from build123d import *

# Parameters (mm, degrees)
SKETCH3_R           = 48
BOSS_EXTRUDE2_DEPTH = 20
SKETCH4_W           = 25
SKETCH4_H           = 5
SKETCH4_H_2         = 10
BOSS_EXTRUDE4_DEPTH = 5
SKETCH5_W           = 20
SKETCH5_H           = 7
BOSS_EXTRUDE5_DEPTH = 6
SKETCH6_W           = 24
SKETCH6_H           = 19
BOSS_EXTRUDE6_DEPTH = 19
SKETCH7_R           = 7.15
CUT_EXTRUDE1_DEPTH  = 28
SKETCH8_W           = 3.5
SKETCH8_H           = 19
SKETCH8_W_2         = 7
CUT_EXTRUDE2_DEPTH  = 19


with BuildPart() as part:
    # Sketch3 → Boss-Extrude2 (new body)
    with BuildSketch(Plane(origin=(0, 0, 0), x_dir=(1, 0, 0), z_dir=(0, 1, 0))):
        with Locations(Location((0, 0, 0), (0, 0, 270))):
            Circle(SKETCH3_R)
    extrude(amount=BOSS_EXTRUDE2_DEPTH)

    # Sketch4 → Boss-Extrude4 (add)
    with BuildSketch(Plane(origin=(0, 20, 0), x_dir=(1, 0, 0), z_dir=(0, 1, 0))):
        with Locations((-19.905756196, -7.187203126)):
            Rectangle(SKETCH4_W, SKETCH4_H)
        with Locations((-19.905756196, -12.187203126)):
            Rectangle(SKETCH4_W, SKETCH4_H)
        with Locations((19.905756196, -9.687203126)):
            Rectangle(SKETCH4_W, SKETCH4_H_2)
    extrude(amount=BOSS_EXTRUDE4_DEPTH)

    # Sketch5 → Boss-Extrude5 (add)
    with BuildSketch(Plane(origin=(0, 25, 0), x_dir=(1, 0, 0), z_dir=(0, 1, 0))):
        with Locations((19.905756196, -9.687203126)):
            Rectangle(SKETCH5_W, SKETCH5_H)
        with Locations((-19.905756196, -9.687203126)):
            Rectangle(SKETCH5_W, SKETCH5_H)
    extrude(amount=BOSS_EXTRUDE5_DEPTH)

    # Sketch6 → Boss-Extrude6 (add)
    with BuildSketch(Plane(origin=(0, 20, 0), x_dir=(1, 0, 0), z_dir=(0, 1, 0))):
        with Locations((0, -36.5)):
            Rectangle(SKETCH6_W, SKETCH6_H)
        with Locations((0, 36.5)):
            Rectangle(SKETCH6_W, SKETCH6_H)
    extrude(amount=BOSS_EXTRUDE6_DEPTH)

    # Sketch7 → Cut-Extrude1 (cut)
    with BuildSketch(Plane(origin=(12, 0, 0), x_dir=(0, 0, -1), z_dir=(1, 0, 0))):
        with Locations((-36.5, 27.5)):
            Circle(SKETCH7_R)
        with Locations(Location((36.5, 27.5, 0), (0, 0, 180))):
            Circle(SKETCH7_R)
    extrude(amount=-CUT_EXTRUDE1_DEPTH, mode=Mode.SUBTRACT)

    # Sketch8 → Cut-Extrude2 (cut)
    with BuildSketch(Plane(origin=(0, 39, 0), x_dir=(1, 0, 0), z_dir=(0, 1, 0))):
        with Locations((-1.75, -36.5)):
            Rectangle(SKETCH8_W, SKETCH8_H)
        with Locations((1.75, -36.5)):
            Rectangle(SKETCH8_W, SKETCH8_H)
        with Locations((0, 36.5)):
            Rectangle(SKETCH8_W_2, SKETCH8_H)
    extrude(amount=-CUT_EXTRUDE2_DEPTH, mode=Mode.SUBTRACT)


solid = part.part
Can you work these out from the model? Positions are in its coordinate system, mm. A direction names the side the tool comes from. Coordinates: 2 decimals unless noted, no trailing zeros. Order: outer loops, then holes, each group sorted by start corner. A loop starts at its lowest first (then second) coordinate and runs counter-clockwise, first axis right, second up. Notation, with made-up numbers: M 14,-0.5 L 49,-0.5 A15 cw 49,19.5 Z; hole C 41.5,-3.75 d4. An arc over 180 degrees is marked long. Answer as CSV lines item,"result".
(1) Suppose I cut it at C-C on y = 27.5. Count the separate pieces of the cut face and the enclosed holes in it, plus the area to 3 significant figures.
Geometry check:
separate pieces,"10"
enclosed holes,"0"
area,"440 mm^2"
(2) Suppose I cut it at A-A on z = 34. Please give me the cut outline in (x, y), plus the area to 3 significant figures.
Geometry check:
outline,"M -33.88,0 L 33.88,0 L 33.88,20 L 12,20 L 12,20.8 L 3.5,20.8 L 3.5,20 L -3.5,20 L -3.5,20.8 L -12,20.8 L -12,20 L -33.88,20 Z; M -12,34.2 L -3.5,34.2 L -3.5,39 L -12,39 Z; M 3.5,34.2 L 12,34.2 L 12,39 L 3.5,39 Z"
area,"1,450 mm^2"
(3) I'm going to push flat-ended pins straight in: pin 1 (2 mm diameter, centred on x = -19, z = 8.5, fed in from +Y); pin 2 (1.5 mm diameter, centred on x = 1.5, y = 25.5, fed in from +Z); pin 3 (4 mm diameter, centred on x = 24, y = 23.5, fed in from -Z); pin 4 (2.5 mm diameter, centred on y = 22, z = 12, fed in from -X). Where does each tip first touch, or does it pass through?
Geometry check:
pin 1,"y = 31"
pin 2,"through"
pin 3,"z = 4.69"
pin 4,"x = -32.41"
(4) Suppose I cut it at B-B on x = 5.5. Please give me the cut outline in (y, z), plus the area to 3 significant figures.
Geometry check:
outline,"M 0,-47.68 L 20,-47.68 L 20,-46 L 39,-46 L 39,-27 L 20,-27 L 20,27 L 39,27 L 39,46 L 20,46 L 20,47.68 L 0,47.68 Z; hole C 27.5,-36.5 d14.3; hole C 27.5,36.5 d14.3"
area,"2,310 mm^2"
(5) On a 3-axis mill with a long thin cutter (end or side, diameter ignored), from which of +Z, -Z, +X, -X, +Y, -Y can I reach the whole of each face in a straight line? I mean faces 1 (the flat face through (-20, 22, 4.687)), 2 (the flat face through (8, 29, -46)), 3 (the flat face through (-29.906, 28, 10)). Say none if no direction works.
Geometry check:
face 1,"+X, -X, +Y"
face 2,"-Z, +X, -X, +Y"
face 3,"+Z, -Z, -X, +Y"
(6) Please list where these lines run through material, in increasing order: L1, parallel to Z at x = -9, y = 27; L2, parallel to Y at x = 6, z = -36.5; L3, parallel to X at y = 29, z = 10.
Geometry check:
L1,"-46 to -43.63, -29.37 to -27, 27 to 29.37, 43.63 to 46"
L2,"0 to 20.35, 34.65 to 39"
L3,"-29.91 to -9.91, 9.91 to 29.91"
(7) Suppose I cut it at D-D on y = 7. Please give me the cut outline in (x, z), plus the area to 3 significant figures.
Geometry check:
outline,"C 0,0 d96"
area,"7,240 mm^2"
(8) If we mould it in two halves opening along X, with no side actions, what happens to faces 4 (the flat face through (20, 25, 14)), 5 (the flat face through (32.406, 22, 10)), 6 (the flat face through (20, 22, 14.687))? For each: released by +X, released by -X, zero draft, split by the parting line, or undercut.
Geometry check:
face 4,"undercut"
face 5,"released by +X"
face 6,"zero draft"
